Build history of the part. All positions in model axes, mm. Face numbers are marked on the shaded views. Round coordinates to 2 decimals unless told otherwise and drop trailing zeros. Order: outer loops, then holes, each group sorted by start corner. A loop starts at its lowest first (then second) coordinate and runs counter-clockwise, first axis right, second up. Notation, with made-up numbers: M 56,-1 L 61,-1 A26 ccw 61,31 Z; hole C 59.25,81 d9. An arc over 180 degrees is marked long. One line per item, written item: value. Start each with the question number.
Item 1: Band-saw the part on D-D, the plane y = 67.25. Write the cut outline in (x, z), then the cut area to 3 significant figures.
Item 2: Probe L1, parallel to Y at x = 107.5, z = 0.45; L2, parallel to X at y = 62.5, z = 2.55; L3, parallel to X at y = 62, z = 0.95. List the from-to ranges inside material, lowest first.
Item 3: Band-saw the part on B-B, the plane y = 63. Write the cut outline in (x, z), then the cut area to 3 significant figures.
Item 4: Band-saw the part on A-A, the plane x = 106.25. Write the cut outline in (y, z), then the cut area to 3 significant figures.
Item 5: Band-saw the part on C-C, the plane z = -1.45. Write the cut outline in (x, y), then the cut area to 3 significant figures.
Item 6: Two-plate mould, pull along Y, no slides. Class the marked faces 1, 2 and 3: +Y half, -Y half, draft (parallel to the pull), parting line (faces both ways), or undercut.
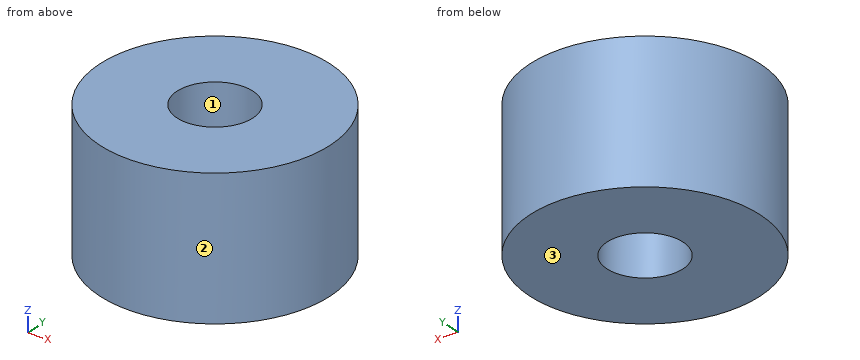
```python
from build123d import *

# Parameters (mm, degrees)
SKETCH_1_R          = 1.65
EXTRUDE_1_DEPTH     = 3
FILLET_1_R          = 4
FILLET_2_R          = 2
SKETCH_2_R          = 32.383706152
SKETCH_2_R_2        = 5
CUT_EXTRUDE_1_DEPTH = 10


with BuildPart() as part:
    # ｽｹｯﾁ1 → ﾎﾞｽ - 押し出し1 (new, symmetric)
    with BuildSketch(Plane.XY):
        Polygon((103.035796932, 67.586451292), (103.035796932, 78.476037139), (111.915158488, 78.476037139), (111.915158488, 67.586451292), (122.804744336, 67.586451292), (122.804744336, 58.707089735), (111.915158488, 58.707089735), (111.915158488, 47.817503888), (103.035796932, 47.817503888), (103.035796932, 58.707089735), (92.146211085, 58.707089735), (92.146211085, 67.586451292), align=None)
        with Locations((107.47547771, 63.146770513)):
            Circle(SKETCH_1_R, mode=Mode.SUBTRACT)
    extrude(amount=EXTRUDE_1_DEPTH, both=True)

    # ﾌｨﾚｯﾄ1
    fillet_1_edges = [part.edges().sort_by_distance(p)[0] for p in [
        (122.804744336, 67.586451292, 0),
        (111.915158488, 47.817503888, 0),
        (92.146211085, 58.707089735, 0),
        (103.035796932, 78.476037139, 0),
    ]]
    fillet(fillet_1_edges, radius=FILLET_1_R)

    # ﾌｨﾚｯﾄ2
    fillet_2_edges = [part.edges().sort_by_distance(p)[0] for p in [
        (111.915158488, 67.586451292, 0),
        (111.915158488, 58.707089735, 0),
        (103.035796932, 58.707089735, 0),
        (103.035796932, 67.586451292, 0),
    ]]
    fillet(fillet_2_edges, radius=FILLET_2_R)

    # ｽｹｯﾁ2 → ｶｯﾄ - 押し出し1 (cut)
    with BuildSketch(Plane.XY.offset(3)):
        with Locations((107.47547771, 63.146770513)):
            Circle(SKETCH_2_R)
        with BuildLine():
            Line((103.035796932, 47.817503888), (107.915158488, 47.817503888))
            ThreePointArc((107.915158488, 47.817503888), (110.743585613, 48.989076763), (111.915158488, 51.817503888))
            Line((111.915158488, 51.817503888), (111.915158488, 56.707089735))
            ThreePointArc((111.915158488, 56.707089735), (112.500944926, 58.121303298), (113.915158488, 58.707089735))
            Line((113.915158488, 58.707089735), (122.804744336, 58.707089735))
            Line((122.804744336, 58.707089735), (122.804744336, 63.586451292))
            ThreePointArc((122.804744336, 63.586451292), (121.63317146, 66.414878416), (118.804744336, 67.586451292))
            Line((118.804744336, 67.586451292), (113.915158488, 67.586451292))
            ThreePointArc((113.915158488, 67.586451292), (112.500944926, 68.172237729), (111.915158488, 69.586451292))
            Line((111.915158488, 69.586451292), (111.915158488, 78.476037139))
            Line((111.915158488, 78.476037139), (107.035796932, 78.476037139))
            ThreePointArc((107.035796932, 78.476037139), (104.207369807, 77.304464263), (103.035796932, 74.476037139))
            Line((103.035796932, 74.476037139), (103.035796932, 69.586451292))
            ThreePointArc((103.035796932, 69.586451292), (102.450010495, 68.172237729), (101.035796932, 67.586451292))
            Line((101.035796932, 67.586451292), (92.146211085, 67.586451292))
            Line((92.146211085, 67.586451292), (92.146211085, 62.707089735))
            ThreePointArc((92.146211085, 62.707089735), (93.31778396, 59.87866261), (96.146211085, 58.707089735))
            Line((96.146211085, 58.707089735), (101.035796932, 58.707089735))
            ThreePointArc((101.035796932, 58.707089735), (102.450010495, 58.121303298), (103.035796932, 56.707089735))
            Line((103.035796932, 56.707089735), (103.035796932, 47.817503888))
        make_face(mode=Mode.SUBTRACT)
        with BuildLine():
            Line((103.035796932, 56.707089735), (103.035796932, 47.817503888))
            Line((103.035796932, 47.817503888), (107.915158488, 47.817503888))
            ThreePointArc((107.915158488, 47.817503888), (110.743585613, 48.989076763), (111.915158488, 51.817503888))
            Line((111.915158488, 51.817503888), (111.915158488, 56.707089735))
            ThreePointArc((111.915158488, 56.707089735), (112.500944926, 58.121303298), (113.915158488, 58.707089735))
            Line((113.915158488, 58.707089735), (122.804744336, 58.707089735))
            Line((122.804744336, 58.707089735), (122.804744336, 63.586451292))
            ThreePointArc((122.804744336, 63.586451292), (121.63317146, 66.414878416), (118.804744336, 67.586451292))
            Line((118.804744336, 67.586451292), (113.915158488, 67.586451292))
            ThreePointArc((113.915158488, 67.586451292), (112.500944926, 68.172237729), (111.915158488, 69.586451292))
            Line((111.915158488, 69.586451292), (111.915158488, 78.476037139))
            Line((111.915158488, 78.476037139), (107.035796932, 78.476037139))
            ThreePointArc((107.035796932, 78.476037139), (104.207369807, 77.304464263), (103.035796932, 74.476037139))
            Line((103.035796932, 74.476037139), (103.035796932, 69.586451292))
            ThreePointArc((103.035796932, 69.586451292), (102.450010495, 68.172237729), (101.035796932, 67.586451292))
            Line((101.035796932, 67.586451292), (92.146211085, 67.586451292))
            Line((92.146211085, 67.586451292), (92.146211085, 62.707089735))
            ThreePointArc((92.146211085, 62.707089735), (93.31778396, 59.87866261), (96.146211085, 58.707089735))
            Line((96.146211085, 58.707089735), (101.035796932, 58.707089735))
            ThreePointArc((101.035796932, 58.707089735), (102.450010495, 58.121303298), (103.035796932, 56.707089735))
        make_face()
        with Locations((107.47547771, 63.146770513)):
            Circle(SKETCH_2_R_2, mode=Mode.SUBTRACT)
    extrude(amount=-CUT_EXTRUDE_1_DEPTH, mode=Mode.SUBTRACT)


solid = part.part
```
Output:
1. outline: M 104.62,-3 L 110.33,-3 L 110.33,3 L 104.62,3 Z
1. area: 34.3 mm²
2. L1: y = 58.15 to 61.5, 64.8 to 68.15
2. L2: x = 102.52 to 105.96, 108.99 to 112.43
2. L3: x = 102.61 to 106.29, 108.66 to 112.34
3. outline: M 102.48,-3 L 105.83,-3 L 105.83,3 L 102.48,3 Z; M 109.12,-3 L 112.47,-3 L 112.47,3 L 109.12,3 Z
3. area: 40.3 mm²
4. outline: M 58.3,-3 L 62.04,-3 L 62.04,3 L 58.3,3 Z; M 64.25,-3 L 67.99,-3 L 67.99,3 L 64.25,3 Z
4. area: 44.9 mm²
5. outline: C 107.48,63.15 d10; hole C 107.48,63.15 d3.3
5. area: 70.0 mm²
6. face 1: undercut
6. face 2: parting line
6. face 3: draft
